```python
from build123d import *

# Parameters (mm, degrees)
CROQUIS1_W                   = 45
CROQUIS1_H                   = 500
CROQUIS1_W_2                 = 500
CROQUIS1_H_2                 = 45
CROQUIS1_R                   = 45
SALIENTE_EXTRUIR1_DEPTH      = 40
CROQUIS2_R                   = 42.35
SALIENTE_EXTRUIR2_DEPTH      = 200
CROQUIS3_R                   = 39.35
CORTAR_EXTRUIR1_DEPTH        = 200
SALIENTE_EXTRUIR3_DEPTH      = 4
SALIENTE_EXTRUIR3_DEPTH_BACK = 200
CROQUIS4_R                   = 39.35
CROQUIS4_R_2                 = 36.35
CROQUIS6_W                   = 121.5
CROQUIS6_H                   = 101
SALIENTE_EXTRUIR4_DEPTH      = 4


with BuildPart() as part:
    # Croquis1 → Saliente-Extruir1 (new body)
    with BuildSketch(Plane(origin=(0, 0, 0), x_dir=(1, 0, 0), z_dir=(0, 1, 0))):
        with Locations((22.5, -295)):
            Rectangle(CROQUIS1_W, CROQUIS1_H)
        with Locations((-22.5, -295)):
            Rectangle(CROQUIS1_W, CROQUIS1_H)
        with Locations((295, -22.5)):
            Rectangle(CROQUIS1_W_2, CROQUIS1_H_2)
        with Locations((295, 22.5)):
            Rectangle(CROQUIS1_W_2, CROQUIS1_H_2)
        with Locations((-295, 22.5)):
            Rectangle(CROQUIS1_W_2, CROQUIS1_H_2)
        with Locations((-295, -22.5)):
            Rectangle(CROQUIS1_W_2, CROQUIS1_H_2)
        with BuildLine():
            Line((-45, -45), (0, -45))
            ThreePointArc((0, -45), (-31.819805153, -31.819805153), (-45, 0))
            Line((-45, 0), (-45, -45))
        make_face()
        with BuildLine():
            ThreePointArc((0, 45), (31.819805153, 31.819805153), (45, 0))
            Line((45, 0), (45, 45))
            Line((45, 45), (0, 45))
        make_face()
        with BuildLine():
            ThreePointArc((-45, 0), (-31.819805153, 31.819805153), (0, 45))
            Line((0, 45), (-45, 45))
            Line((-45, 45), (-45, 0))
        make_face()
        with Locations((-22.5, 295)):
            Rectangle(CROQUIS1_W, CROQUIS1_H)
        with Locations((22.5, 295)):
            Rectangle(CROQUIS1_W, CROQUIS1_H)
        with BuildLine():
            Line((45, -45), (45, 0))
            ThreePointArc((45, 0), (31.819805153, -31.819805153), (0, -45))
            Line((0, -45), (45, -45))
        make_face()
        Circle(CROQUIS1_R)
    extrude(amount=SALIENTE_EXTRUIR1_DEPTH)

    # Croquis2 → Saliente-Extruir2 (add)
    with BuildSketch(Plane(origin=(0, 40, 0), x_dir=(1, 0, 0), z_dir=(0, 1, 0))):
        with Locations(Location((0, 0, 0), (0, 0, 270))):
            Circle(CROQUIS2_R)
    extrude(amount=SALIENTE_EXTRUIR2_DEPTH)

    # Croquis3 → Cortar-Extruir1 (cut)
    with BuildSketch(Plane(origin=(0, 240, 0), x_dir=(1, 0, 0), z_dir=(0, 1, 0))):
        with Locations(Location((0, 0, 0), (0, 0, 270))):
            Circle(CROQUIS3_R)
    extrude(amount=-CORTAR_EXTRUIR1_DEPTH, mode=Mode.SUBTRACT)

    # Croquis4 → Saliente-Extruir3 (add, two sides: drawn at the far end of the back side and taken through both)
    with BuildSketch(Plane(origin=(0, 240, 0), x_dir=(1, 0, 0), z_dir=(0, 1, 0)).offset(-SALIENTE_EXTRUIR3_DEPTH_BACK)):
        with Locations(Location((0, 0, 0), (0, 0, 270))):
            Circle(CROQUIS4_R)
        with Locations(Location((0, 0, 0), (0, 0, 270))):
            Circle(CROQUIS4_R_2, mode=Mode.SUBTRACT)
    extrude(amount=SALIENTE_EXTRUIR3_DEPTH + SALIENTE_EXTRUIR3_DEPTH_BACK)

    # Croquis6 → Saliente-Extruir4 (add)
    with BuildSketch(Plane(origin=(0, 240, 0), x_dir=(1, 0, 0), z_dir=(0, 1, 0))):
        Rectangle(CROQUIS6_W, CROQUIS6_H)
    extrude(amount=SALIENTE_EXTRUIR4_DEPTH)


solid = part.part
```
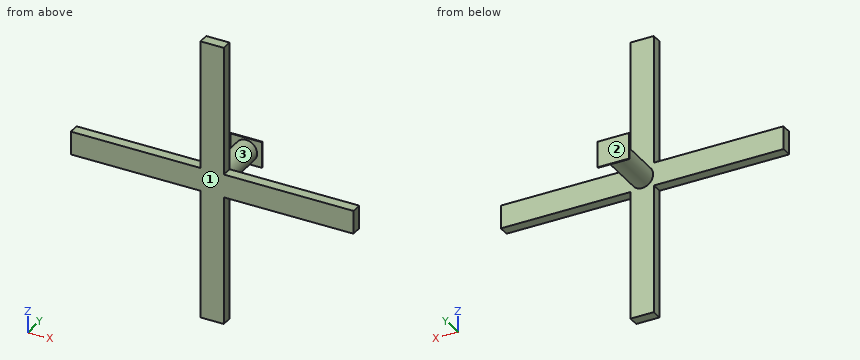
Geometry: final body of the model. Coordinates: model frame, mm. Face numbers are marked on the shaded views. Give positions to 0.01 mm unless a question says otherwise; leave off trailing zeros. Write each loop counter-clockwise with the first axis right and the second up, starting at its lowest first coordinate (ties: lowest second). Pieces come first, ordered by that corner, then holes.
1. Section query C-C, the plane y = 205.5. Return loops of the section in (x, z), then the cut area to 3 significant figures.
2. Section query B-B, the plane x = 0. Return loops of the section in (y, z), then the cut area to 3 significant figures.
3. Draft query along Y for the marked faces 1, 2 and 3. Return one class per face: released by +Y, released by -Y, zero draft, split by the parting line, or undercut.
4. Pin query (flat end, axial travel): P1, Ø20, axis at x = -179, y = 22, coming from the -Z side; P2, Ø1.2, axis at x = -4, y = 242, coming from the -Z side; P3, Ø4.5, axis at x = 13.5, y = 242, coming from the +Z side. Return the tip coordinate at first contact, or that it passes through.
5. Section query A-A, the plane z = 0. Return loops of the section in (x, y).
6. Line query: probe 1 along X at (y, z) = (120.5, 0); probe 2 along Y at (x, z) = (-30, 308); probe 3 along Z at (x, y) = (62, 30.5). Output: solid intervals per line, ascending.
7. Section query D-D, the plane z = -448. Return loops of the section in (x, y), then the cut area to 3 significant figures.
Computed:
1. outline: circle Ø84.7 at (0, 0); hole circle Ø72.7 at (0, 0)
1. area: 1,480 mm2
2. outline: (0, -545) - (40, -545) - (40, -42.35) - (240, -42.35) - (240, -50.5) - (244, -50.5) - (244, 50.5) - (240, 50.5) - (240, 42.35) - (40, 42.35) - (40, 545) - (0, 545) - close; hole (40, -36.35) - (240, -36.35) - (240, 36.35) - (40, 36.35) - close
2. area: 46,400 mm2
3. face 1: released by -Y
3. face 2: released by +Y
3. face 3: undercut
4. P1: stops at z = -45
4. P2: stops at z = -50.5
4. P3: stops at z = 50.5
5. outline: (-545, 0) - (545, 0) - (545, 40) - (42.35, 40) - (42.35, 240) - (60.75, 240) - (60.75, 244) - (-60.75, 244) - (-60.75, 240) - (-42.35, 240) - (-42.35, 40) - (-545, 40) - close; hole (-36.35, 40) - (36.35, 40) - (36.35, 240) - (-36.35, 240) - close
6. probe 1: x = -42.35 to -36.35, 36.35 to 42.35
6. probe 2: y = 0 to 40
6. probe 3: z = -45 to 45
7. outline: (-45, 0) - (45, 0) - (45, 40) - (-45, 40) - close
7. area: 3,600 mm2
